The model under review builds one solid part; all positions refer to its coordinate system, in mm. Coordinates: 2 decimals unless noted, no trailing zeros. Write each loop counter-clockwise with the first axis right and the second up, starting at its lowest first coordinate (ties: lowest second). Pieces come first, ordered by that corner, then holes.
1) For P1, Ø12, axis at y = 443, z = -626, coming from the -X side; P2, Ø15, axis at x = -380.5, z = -448, coming from the -Y side; P3, Ø25, axis at x = 1059.5, y = 291, coming from the +Z side, all flat-tipped, find the tip position at first contact; note any pin that passes through.
2) Add section C-C, the plane z = -477. State the section outline as (x, y) points.
3) For line 1 (Y direction, x = -36.5, z = -185); line 2 (X direction, y = 740, z = -43); line 3 (Z direction, x = -19, y = -93.5), list the stretches that pass through material, from the lowest coordinate up.
4) Add section B-B, the plane x = 239. State the section outline as (y, z) points.
5) Add section A-A, the plane y = 822.5. Give the number of separate pieces and of enclosed holes in the cut face, then the cut area to 3 significant figures.
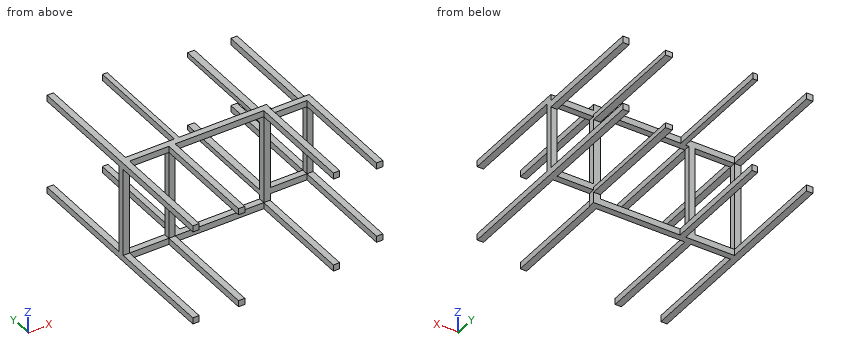
from build123d import *

# Parameters (mm, degrees)
CROQUIS1_W              = 700
CROQUIS1_H              = 700
CROQUIS1_W_2            = 287.203756055
CROQUIS1_H_2            = 547.555321307
CROQUIS1_W_3            = 311.038292855
SALIENTE_EXTRUIR1_DEPTH = 50
CROQUIS2_W              = 50
CROQUIS2_H              = 50
SALIENTE_EXTRUIR2_DEPTH = 850
CROQUIS3_W              = 50
CROQUIS3_H              = 50
CROQUIS3_H_2            = 52.444678691
CROQUIS3_W_2            = 44.735144292
CROQUIS3_W_3            = 37.538527074
CROQUIS3_W_4            = 54.044332967
CROQUIS3_H_3            = 39.518840668
CROQUIS3_W_5            = 54.044332968
CROQUIS3_H_4            = 39.951892275
SALIENTE_EXTRUIR3_DEPTH = 879.0597314
CROQUIS4_W              = 50
CROQUIS4_H              = 50
SALIENTE_EXTRUIR4_DEPTH = 850


with BuildPart() as part:
    # Croquis1 → Saliente-Extruir1 (new body)
    with BuildSketch(Plane(origin=(0, 0, 0), x_dir=(1, 0, 0), z_dir=(0, 1, 0))):
        Polygon((-45.955667033, -50), (754.044332967, -50), (754.044332967, 0), (1091.248089022, 0), (1091.248089022, 52.444678693), (1091.248089022, 647.555321307), (754.044332967, 647.555321307), (754.044332967, 750), (-45.955667033, 750), (-411.038292855, 750), (-411.038292855, -50), align=None)
        with Locations((350, 350)):
            Rectangle(CROQUIS1_W, CROQUIS1_H, mode=Mode.SUBTRACT)
        with Locations((897.646210995, 323.777660653)):
            Rectangle(CROQUIS1_W_2, CROQUIS1_H_2, mode=Mode.SUBTRACT)
        with Locations((-205.519146428, 350)):
            Rectangle(CROQUIS1_W_3, CROQUIS1_H, mode=Mode.SUBTRACT)
    extrude(amount=SALIENTE_EXTRUIR1_DEPTH)

    # Croquis2 → Saliente-Extruir2 (add)
    with BuildSketch(Plane.XZ):
        with Locations((-25, 25)):
            Rectangle(CROQUIS2_W, CROQUIS2_H)
        with Locations((725, 25)):
            Rectangle(CROQUIS2_W, CROQUIS2_H)
        with Locations((725, -725)):
            Rectangle(CROQUIS2_W, CROQUIS2_H)
        with Locations((-25, -725)):
            Rectangle(CROQUIS2_W, CROQUIS2_H)
    extrude(amount=SALIENTE_EXTRUIR2_DEPTH)

    # Croquis3 → Saliente-Extruir3 (add)
    with BuildSketch(Plane(origin=(0, 50, 0), x_dir=(1, 0, 0), z_dir=(0, 1, 0))):
        with Locations((-386.038292855, 725)):
            Rectangle(CROQUIS3_W, CROQUIS3_H)
        with Locations((1066.248089022, 622.555321307)):
            Rectangle(CROQUIS3_W, CROQUIS3_H)
        with Locations((1066.248089022, 76.222339346)):
            Rectangle(CROQUIS3_W, CROQUIS3_H_2)
        with Locations((-386.038292855, -25)):
            Rectangle(CROQUIS3_W, CROQUIS3_H)
        with Locations((47.209644204, 725)):
            Rectangle(CROQUIS3_W_2, CROQUIS3_H)
        with Locations((45.029305303, -25)):
            Rectangle(CROQUIS3_W_3, CROQUIS3_H)
        with Locations((727.022166484, 54.312727654)):
            Rectangle(CROQUIS3_W_4, CROQUIS3_H_3)
        with Locations((727.022166484, 645.903798151)):
            Rectangle(CROQUIS3_W_5, CROQUIS3_H_4)
    extrude(amount=SALIENTE_EXTRUIR3_DEPTH)

    # Croquis4 → Saliente-Extruir4 (add)
    with BuildSketch(Plane.XZ):
        with Locations((-386.038292855, 25)):
            Rectangle(CROQUIS4_W, CROQUIS4_H)
        with Locations((-386.038292855, -725)):
            Rectangle(CROQUIS4_W, CROQUIS4_H)
        with Locations((1066.248089022, -622.555321307)):
            Rectangle(CROQUIS4_W, CROQUIS4_H)
        with Locations((1066.248089022, -25)):
            Rectangle(CROQUIS4_W, CROQUIS4_H)
    extrude(amount=SALIENTE_EXTRUIR4_DEPTH)


solid = part.part
Geometry results:
1. P1: stops at x = 700
1. P2: stops at y = 0
1. P3: stops at z = -50
2. outline: (-411.04, 0) - (-361.04, 0) - (-361.04, 50) - (-411.04, 50) - close; (-50, 0) - (0, 0) - (0, 50) - (-50, 50) - close; (700, 0) - (754.04, 0) - (754.04, 50) - (700, 50) - close; (1041.25, 0) - (1091.25, 0) - (1091.25, 50) - (1041.25, 50) - close
3. line 1: y = 0 to 50
3. line 2: x = 700 to 754.04
3. line 3: z = -750 to -700, 0 to 50
4. outline: (0, -750) - (50, -750) - (50, -700) - (0, -700) - close; (0, 0) - (50, 0) - (50, 50) - (0, 50) - close
5. separate pieces: 8
5. enclosed holes: 0
5. area: 18,500 mm2
